from build123d import *

# Parameters (mm, degrees)
F0_R         = 5
F1_DEPTH     = 2
F2_SIZE      = 1.99999
F3_T1_DEPTH  = 34.8509927222
F3_T3_DEPTH  = 34.8509927222
F3_T5_DEPTH  = 34.8509927222
F3_T7_DEPTH  = 34.8509927222
F3_T9_DEPTH  = 34.8509927222
F3_T11_DEPTH = 34.8509927222
F3_T13_DEPTH = 34.8509927222
F3_T15_DEPTH = 34.8509927222


# Not quite as in the source:
# - a fillet or chamfer that OpenCascade refuses, or shapes differently, is made with other operations: its cross-section is extruded or revolved along the edge and cut away or added
# - a fillet or chamfer is up to 0.001 mm smaller than in the source, because OpenCascade refuses the exact size


with BuildPart() as f1:
    # F0 (on Top) → F1 (new body, symmetric)
    with BuildSketch(Plane.XY):
        with BuildLine():
            ThreePointArc((17.093492914, -3.75), (17.3980764166, -1.8859843591), (17.5, 0))
            ThreePointArc((17.5, 0), (17.3980764166, 1.8859843591), (17.093492914, 3.75))
            ThreePointArc((17.093492914, 3.75), (12.3743686708, 12.3743686708), (3.75, 17.093492914))
            ThreePointArc((3.75, 17.093492914), (0, 17.5), (-3.75, 17.093492914))
            ThreePointArc((-3.75, 17.093492914), (-12.3743686708, 12.3743686708), (-17.093492914, 3.75))
            ThreePointArc((-17.093492914, 3.75), (-17.5, 0), (-17.093492914, -3.75))
            ThreePointArc((-17.093492914, -3.75), (-12.3743686708, -12.3743686708), (-3.75, -17.093492914))
            ThreePointArc((-3.75, -17.093492914), (0, -17.5), (3.75, -17.093492914))
            ThreePointArc((3.75, -17.093492914), (12.3743686708, -12.3743686708), (17.093492914, -3.75))
        make_face()
        Circle(F0_R, mode=Mode.SUBTRACT)
        with BuildLine():
            ThreePointArc((-17.093492914, -3.75), (-17.5, 0), (-17.093492914, 3.75))
            Line((-17.093492914, 3.75), (-27.093492914, 3.75))
            Line((-27.093492914, 3.75), (-27.093492914, -3.75))
            Line((-27.093492914, -3.75), (-17.093492914, -3.75))
        make_face()
        Polygon((-27.093492914, -3.75), (-27.093492914, 3.75), (-27.093492914, 8.75), (-52.093492914, 0), (-27.093492914, -8.75), align=None)
        with BuildLine():
            ThreePointArc((-3.75, 17.093492914), (0, 17.5), (3.75, 17.093492914))
            Line((3.75, 17.093492914), (3.75, 27.093492914))
            Line((3.75, 27.093492914), (-3.75, 27.093492914))
            Line((-3.75, 27.093492914), (-3.75, 17.093492914))
        make_face()
        Polygon((-3.75, 27.093492914), (3.75, 27.093492914), (8.75, 27.093492914), (0, 52.093492914), (-8.75, 27.093492914), align=None)
        Polygon((27.093492914, 8.75), (27.093492914, 3.75), (27.093492914, -3.75), (27.093492914, -8.75), (52.093492914, 0), align=None)
        Polygon((8.75, -27.093492914), (3.75, -27.093492914), (-3.75, -27.093492914), (-8.75, -27.093492914), (0, -52.093492914), align=None)
        with BuildLine():
            Line((3.75, -27.093492914), (3.75, -17.093492914))
            ThreePointArc((3.75, -17.093492914), (0, -17.5), (-3.75, -17.093492914))
            Line((-3.75, -17.093492914), (-3.75, -27.093492914))
            Line((-3.75, -27.093492914), (3.75, -27.093492914))
        make_face()
        with BuildLine():
            ThreePointArc((17.093492914, 3.75), (17.3980764166, 1.8859843591), (17.5, 0))
            ThreePointArc((17.5, 0), (17.3980764166, -1.8859843591), (17.093492914, -3.75))
            Line((17.093492914, -3.75), (27.093492914, -3.75))
            Line((27.093492914, -3.75), (27.093492914, 3.75))
            Line((27.093492914, 3.75), (17.093492914, 3.75))
        make_face()
    extrude(amount=F1_DEPTH, both=True)

    # F2 (size 2 in the source; OpenCascade refuses exactly that, so slightly less here)
    f2_edges = [f1.edges().sort_by_distance(p)[0] for p in [
        (4.375, -39.593493, 2),
        (-4.375, -39.593493, 2),
        (4.375, -39.593493, -2),
        (-4.375, -39.593493, -2),
        (39.593493, -4.375, -2),
        (39.593493, -4.375, 2),
        (39.593493, 4.375, 2),
        (-39.593493, -4.375, 2),
        (-39.593493, -4.375, -2),
        (-4.375, 39.593493, 2),
        (4.375, 39.593493, 2),
        (39.593493, 4.375, -2),
        (4.375, 39.593493, -2),
        (-39.593493, 4.375, 2),
        (-39.593493, 4.375, -2),
        (-4.375, 39.593493, -2),
    ]]
    chamfer(f2_edges, length=F2_SIZE)

    # F3: chamfer of 2.85 on 16 edges, made by hand

    # F3_s2 → F3_t1 (cut)
    with BuildSketch(Plane(origin=(-16.7962484861, -47.9892813888, 0), x_dir=(0, 0, 1), z_dir=(0.3303504247, 0.9438583564, 0))):
        Polygon((2, 12.3591175097), (-0.0152543264, 17.2243718361), (2, 15.2091175097), align=None)
        Polygon((-2, 12.3591175097), (0.0152543264, 17.2243718361), (-2, 15.2091175097), align=None)
    extrude(amount=F3_T1_DEPTH, mode=Mode.SUBTRACT)

    # F3_s4 → F3_t3 (cut)
    with BuildSketch(Plane(origin=(5.2832082381, -15.0948806803, 0), x_dir=(0, 0, 1), z_dir=(0.3303504247, -0.9438583564, 0))):
        Polygon((2, 12.3591175097), (-0.0152543264, 17.2243718361), (2, 15.2091175097), align=None)
        Polygon((-2, 12.3591175097), (0.0152543264, 17.2243718361), (-2, 15.2091175097), align=None)
    extrude(amount=F3_T3_DEPTH, mode=Mode.SUBTRACT)

    # F3_s6 → F3_t5 (cut)
    with BuildSketch(Plane(origin=(15.0948806803, 5.2832082381, 0), x_dir=(0, 0, 1), z_dir=(0.9438583564, 0.3303504247, 0))):
        Polygon((2, 12.3591175097), (-0.0152543264, 17.2243718361), (2, 15.2091175097), align=None)
        Polygon((-2, 12.3591175097), (0.0152543264, 17.2243718361), (-2, 15.2091175097), align=None)
    extrude(amount=F3_T5_DEPTH, mode=Mode.SUBTRACT)

    # F3_s8 → F3_t7 (cut)
    with BuildSketch(Plane(origin=(47.9892813888, -16.7962484861, 0), x_dir=(0, 0, 1), z_dir=(-0.9438583564, 0.3303504247, 0))):
        Polygon((2, 12.3591175097), (-0.0152543264, 17.2243718361), (2, 15.2091175097), align=None)
        Polygon((-2, 12.3591175097), (0.0152543264, 17.2243718361), (-2, 15.2091175097), align=None)
    extrude(amount=F3_T7_DEPTH, mode=Mode.SUBTRACT)

    # F3_s10 → F3_t9 (cut)
    with BuildSketch(Plane(origin=(-5.2832082381, 15.0948806803, 0), x_dir=(0, 0, 1), z_dir=(-0.3303504247, 0.9438583564, 0))):
        Polygon((2, 12.3591175097), (-0.0152543264, 17.2243718361), (2, 15.2091175097), align=None)
        Polygon((-2, 12.3591175097), (0.0152543264, 17.2243718361), (-2, 15.2091175097), align=None)
    extrude(amount=F3_T9_DEPTH, mode=Mode.SUBTRACT)

    # F3_s12 → F3_t11 (cut)
    with BuildSketch(Plane(origin=(16.7962484861, 47.9892813888, 0), x_dir=(0, 0, 1), z_dir=(-0.3303504247, -0.9438583564, 0))):
        Polygon((-0.0152543264, 17.2243718361), (2, 12.3591175097), (2, 15.2091175097), align=None)
        Polygon((0.0152543264, 17.2243718361), (-2, 12.3591175097), (-2, 15.2091175097), align=None)
    extrude(amount=F3_T11_DEPTH, mode=Mode.SUBTRACT)

    # F3_s14 → F3_t13 (cut)
    with BuildSketch(Plane(origin=(-15.0948806803, -5.2832082381, 0), x_dir=(0, 0, 1), z_dir=(-0.9438583564, -0.3303504247, 0))):
        Polygon((2, 12.3591175097), (-0.0152543264, 17.2243718361), (2, 15.2091175097), align=None)
        Polygon((-2, 12.3591175097), (0.0152543264, 17.2243718361), (-2, 15.2091175097), align=None)
    extrude(amount=F3_T13_DEPTH, mode=Mode.SUBTRACT)

    # F3_s16 → F3_t15 (cut)
    with BuildSketch(Plane(origin=(-47.9892813888, 16.7962484861, 0), x_dir=(0, 0, 1), z_dir=(0.9438583564, -0.3303504247, 0))):
        Polygon((2, 12.3591175097), (-0.0152543264, 17.2243718361), (2, 15.2091175097), align=None)
        Polygon((-2, 12.3591175097), (0.0152543264, 17.2243718361), (-2, 15.2091175097), align=None)
    extrude(amount=F3_T15_DEPTH, mode=Mode.SUBTRACT)


solid = f1.part
Source: CAD feature listing. Evaluate the final solid. Frame: model axes, mm. A direction names the side the tool comes from. Give positions to 0.01 mm unless a question says otherwise; leave off trailing zeros. Write each loop counter-clockwise with the first axis right and the second up, starting at its lowest first coordinate (ties: lowest second). Pieces come first, ordered by that corner, then holes. Notation, with made-up numbers: M 41.5,-36.75 L 98.5,-36.75 A29 cw 98.5,1.25 Z; hole C -27.5,65 d2. An arc over 180 degrees is marked long. Return JSON: item names as keys, results as strings. Group by question number.
1) Cut plane C-C, the plane y = -34. Output: boundary loops of the cut face in (x, z), then the cut area to 3 significant figures.
2) Ray query, L1, parallel to Y at x = 24, z = -0.9; L2, parallel to X at y = 15, z = 0. Return the intervals inside material, ascending.
3) Set-up query: faces 4 (the face through (3.75, 22, 0)), 5 (the face through (-3.75, -22, 0)), 6 (the face through (12.28, -12.47, 0.03)), 7 (the face through (-22, -3.75, 0)), 8 (the face through (22, 3.75, 0)). Return all of +Z, -Z, +X, -X, +Y, -Y with unobstructed straight access to the full face (end or side cutting, diameter ignored); none if empty.
4) Draft query along X for faces 1 (the face through (3.75, -22, 0)), 2 (the face through (-27.093, 6, 0)), 3 (the face through (3, -5, 2)). Return one class per face: released by +X, released by -X, zero draft, split by the parting line, or undercut.
5) Cut plane D-D, the plane x = -35. Output: boundary loops of the cut face in (y, z), then the cut area to 3 significant figures.
6) Cut plane B-B, the plane x = 22. Output: boundary loops of the cut face in (y, z), then the cut area to 3 significant figures.
7) First-contact query: pin 1 Ø1.5 at (y, z) = (41, 0) entering from -X; pin 2 Ø1.2 at (x, z) = (-21.5, -0.5) entering from +Y; pin 3 Ø2 at (y, z) = (-21, 0.5) entering from -X. Flat tips, straight axial feed; report the tip coordinate or a pass-through.
Data:
{
 "1": {"outline": "M -6.31,0 L -1.19,-2 L 1.19,-2 L 6.31,0 L 1.19,2 L -1.19,2 Z", "area": "30.0 mm²"},
 "2": {"L1": "y = -3.75 to 3.75", "L2": "x = -9.01 to 9.01"},
 "3": {"face 4": "+Z, -Z, +X", "face 5": "+Z, -Z, -X", "face 6": "+Z, -Z", "face 7": "+Z, -Z, -Y", "face 8": "+Z, -Z, +Y"},
 "4": {"face 1": "released by +X", "face 2": "undercut", "face 3": "zero draft"},
 "5": {"outline": "M -5.96,0 L -0.84,-2 L 0.84,-2 L 5.96,0 L 0.84,2 L -0.84,2 Z", "area": "27.2 mm²"},
 "6": {"outline": "M -3.75,-2 L 3.75,-2 L 3.75,2 L -3.75,2 Z", "area": "30.0 mm²"},
 "7": {"pin 1": "stops at x = -4.12", "pin 2": "stops at y = 3.75", "pin 3": "stops at x = -3.75"}
}
